from build123d import *

# Parameters (mm, degrees)
EXTRUDE_1_DEPTH     = 6
CUT_EXTRUDE_1_DEPTH = 3.8
CUT_EXTRUDE_2_DEPTH = 49.87803699
SKETCH_3_W          = 18.536502565
SKETCH_3_H          = 15.637579157
CUT_EXTRUDE_3_DEPTH = 4
SKETCH_4_W          = 6
SKETCH_4_H          = 10
EXTRUDE_2_DEPTH     = 19.25
SKETCH_5_R          = 0.85
CUT_EXTRUDE_4_DEPTH = 50.639324129
SKETCH_6_R          = 0.85
CUT_EXTRUDE_5_DEPTH = 6


with BuildPart() as part:
    # 草图1 → 凸台-拉伸1 (new body)
    with BuildSketch(Plane(origin=(0, 0, 0), x_dir=(0, 0, -1), z_dir=(1, 0, 0))):
        Polygon((-25, 5), (25, 5), (25, 3), (48.25, 3), (48.25, -3), (25, -3), (25, -5), (-25, -5), (-25, -3), (-48.25, -3), (-48.25, 3), (-25, 3), align=None)
    extrude(amount=-EXTRUDE_1_DEPTH)

    # 草图1<3> → 切除-拉伸1 (cut)
    with BuildSketch(Plane(origin=(0, 0, 0), x_dir=(0, 0, -1), z_dir=(1, 0, 0))):
        with BuildLine():
            Line((-15.5, 2.25), (15.5, 2.25))
            ThreePointArc((15.5, 2.25), (17.75, 0), (15.5, -2.25))
            Line((15.5, -2.25), (-15.5, -2.25))
            ThreePointArc((-15.5, -2.25), (-17.75, 0), (-15.5, 2.25))
        make_face()
    extrude(amount=-CUT_EXTRUDE_1_DEPTH, mode=Mode.SUBTRACT)

    # 草图1<4> → 切除-拉伸2 (cut, through all)
    with BuildSketch(Plane(origin=(0, 0, 0), x_dir=(0, 0, -1), z_dir=(1, 0, 0))):
        with BuildLine():
            Line((-12.3, 2.25), (12.3, 2.25))
            ThreePointArc((12.3, 2.25), (14.55, 0), (12.3, -2.25))
            Line((12.3, -2.25), (-12.3, -2.25))
            ThreePointArc((-12.3, -2.25), (-14.55, 0), (-12.3, 2.25))
        make_face()
    extrude(amount=-CUT_EXTRUDE_2_DEPTH, mode=Mode.SUBTRACT)

    # 草图3 → 切除-拉伸3 (cut)
    with BuildSketch(Plane(origin=(0, 0, -48.25), x_dir=(-1, 0, 0), z_dir=(0, 0, -1))):
        with Locations((1.626975839, 1.766046581)):
            Rectangle(SKETCH_3_W, SKETCH_3_H)
    extrude(amount=-CUT_EXTRUDE_3_DEPTH, mode=Mode.SUBTRACT)

    # 草图4 → 凸台-拉伸2 (add)
    with BuildSketch(Plane(origin=(0, 0, -25), x_dir=(-1, 0, 0), z_dir=(0, 0, -1))):
        with Locations((3, 0)):
            Rectangle(SKETCH_4_W, SKETCH_4_H)
    extrude(amount=EXTRUDE_2_DEPTH)

    # 草图5 → 切除-拉伸4 (cut, through all)
    with BuildSketch(Plane.XZ.offset(5)):
        with Locations(Location((-2.8, 31, 0), (0, 0, 270))):
            Circle(SKETCH_5_R)
        with Locations(Location((-2.8, -31, 0), (0, 0, 270))):
            Circle(SKETCH_5_R)
    extrude(amount=-CUT_EXTRUDE_4_DEPTH, mode=Mode.SUBTRACT)

    # 草图6 → 切除-拉伸5 (cut)
    with BuildSketch(Plane(origin=(0, 0, -44.25), x_dir=(-1, 0, 0), z_dir=(0, 0, -1))):
        with Locations((3, 0)):
            Circle(SKETCH_6_R)
    extrude(amount=-CUT_EXTRUDE_5_DEPTH, mode=Mode.SUBTRACT)


solid = part.part
For this review, take the finished solid that the model builds, in its own axes (mm). A direction names the side the tool comes from. Give positions to 0.01 mm unless a question says otherwise; leave off trailing zeros. Loops run counter-clockwise (first coordinate to the right, second up) from the corner with the lowest first, then second, coordinate; pieces in that order, holes last.
Item 1: Take a section at D-D, the plane z = -31. State the section outline as (x, y) points.
Item 2: Take a section at A-A, the plane y = 0. State the section outline as (x, z) points, and give its area (3 significant figures).
Item 3: Take a section at C-C, the plane x = -0.95. State the section outline as (y, z) points, and give its area (3 significant figures).
Item 4: Tool access review of faces 1 (the flat face through (-3.8, 0, -16)), 2 (the flat face through (-3, -3, 36)), 3 (the flat face through (-3, 4, 25)): name each direction out of +Z, -Z, +X, -X, +Y, -Y from which nothing blocks a thin tool from reaching the whole face with its end or side.
Item 5: Draft analysis for pull direction Z (two halves, no side actions). For faces 4 (the flat face through (-3, 5, -9)), 5 (the cylindrical face through (-4.88, -0.05, 14.55)), 6 (the flat face through (-3.8, 0, 16)), 7 (the flat face through (-3, 0, 48.25)), state which applies: +Z half, -Z half, draft (parallel to the pull), parting line (faces both ways), or undercut.
Item 6: For line 1 along Z through (x, y) = (-3.1, -1.25); line 2 along Y through (x, z) = (-5.2, 7.5); line 3 along Z through (x, y) = (-5.1, 0.25), list the stretches that pass through material, from the lowest coordinate up.
Item 7: Take a section at B-B, the plane z = 5. State the section outline as (x, y) points.
Item 8: Insertion check: pin 1 (2 mm diameter, centred on y = 1, z = -14, fed in from +X); pin 2 (1 mm diameter, centred on x = -4.5, y = -4, fed in from +Z); pin 3 (3 mm diameter, centred on x = -2, z = 37, fed in from -Y); pin 4 (1.5 mm diameter, centred on y = 2.5, z = -27, fed in from +X). Each pin has a flat end and moves straight along its axis. Give the tip position at first contact, or say it passes through.
Calculated:
1. outline: (-6, -5) - (-3.65, -5) - (-3.65, 5) - (-6, 5) - close; (-1.95, -5) - (0, -5) - (0, 5) - (-1.95, 5) - close
2. outline: (-6, -44.25) - (-3.85, -44.25) - (-3.85, -38.25) - (-2.15, -38.25) - (-2.15, -44.25) - (0, -44.25) - (0, -17.75) - (-3.8, -17.75) - (-3.8, -14.55) - (-6, -14.55) - close; (-6, 14.55) - (-3.8, 14.55) - (-3.8, 17.75) - (0, 17.75) - (0, 48.25) - (-6, 48.25) - close; hole circle Ø1.7 at (-2.8, -31); hole circle Ø1.7 at (-2.8, 31)
2. area: 341 mm2
3. outline: (-5, -44.25) - (5, -44.25) - (5, 25) - (3, 25) - (3, 48.25) - (-3, 48.25) - (-3, 25) - (-5, 25) - close; hole (-2.25, -15.5) arc R2.25 ccw to (2.25, -15.5) - (2.25, 15.5) arc R2.25 ccw to (-2.25, 15.5) - close
3. area: 677 mm2
4. face 1: +X
4. face 2: +Z, +X, -X, -Y
4. face 3: +Z, +X, -X, +Y
5. face 4: draft
5. face 5: undercut
5. face 6: undercut
5. face 7: +Z half
6. line 1: z = -44.25 to -31.8, -30.2 to -17.37, 17.37 to 30.2, 31.8 to 48.25
6. line 2: y = -5 to -2.25, 2.25 to 5
6. line 3: z = -44.25 to -14.54, 14.54 to 48.25
7. outline: (-6, -5) - (0, -5) - (0, -2.25) - (-6, -2.25) - close; (-6, 2.25) - (0, 2.25) - (0, 5) - (-6, 5) - close
8. pin 1: stops at x = -3.8
8. pin 2: stops at z = 25
8. pin 3: stops at y = -3
8. pin 4: stops at x = 0
